Autodesk Inventor part; units mm, degrees
ref_plane "YZ Plane" through (0, 0, 0) normal (1, 0, 0) x (0, 1, 0)
ref_plane "XZ Plane" through (0, 0, 0) normal (0, 1, 0) x (-1, 0, 0)
sketch "Sketch1" plane through (0, 0, 0) normal (0, 0, 1) x (1, 0, 0)
  line L0 (-50, 20) -> (50, 20)
  line L1 (50, 20) -> (50, -20)
  line L2 (50, -20) -> (-50, -20)
  line L3 (-50, -20) -> (-50, 20)
  line L4 (-50, 20) -> (50, -20) construction
  line L5 (50, 20) -> (-50, -20) construction
  point P0 (0, 0)
  dimension "d0" = 100
  dimension "d1" = 40
extrude "Extrusion1" add sketch "Sketch1" along normal blind 20
sketch "Sketch2" plane through (0, 0, 20) normal (0, 0, 1) x (1, 0, 0)
  line L0 (-50, -20) -> (50, -20)
  line L1 (50, -20) -> (50, 20)
  line L2 (50, 20) -> (-50, 20)
  line L3 (-50, 20) -> (-50, -20)
  line L4 (-70, 0) -> (70, 0)
  line L5 (0, -28) -> (0, 28)
  line L6 (50, -20) -> (50, 20)
  line L7 (-50, 17) -> (50, 17)
  line L8 (50, 17) -> (50, 18.5)
  line L9 (50, 18.5) -> (-50, 18.5)
  line L10 (-50, 18.5) -> (-50, 17)
  line L11 (-50, 17) -> (50, 18.5) construction
  line L12 (50, 17) -> (-50, 18.5) construction
  point P0 (0, 0)
  point P1 (0, 17.75)
  dimension "d4" = 1.5
  dimension "d6" = 1.5
extrude "Extrusion2" cut sketch "Sketch2" against normal blind 17 contours L3 L9 L5 L7 | L5 L9 L1 L7
pattern_linear "Rectangular Pattern1" count 13 spacing 3 along (0, -1, 0) of "Extrusion2"
ref_plane "Work Plane1" through (0, 0, 20) normal (0, 0, 1) x (1, 0, 0)
sketch "Sketch4" plane through (0, 0, 20) normal (0, 0, 1) x (1, 0, 0)
  line L0 (0, -28) -> (0, 28)
  line L1 (50, 0.5) -> (50, -1)
  line L2 (50, 20) -> (-50, 20)
  line L3 (-50, -20) -> (50, -20)
  line L4 (-50, -4) -> (-50, -5.5)
  point P0 (0, 0)
  point P1 (44, -13)
  point P2 (-44, -13)
  dimension "d22" = 6
  dimension "d30" = 7
  dimension "d31" = 7
  dimension "d32" = 6
hole "Hole2" at (44, -13, 20) at (-44, -13, 20) direction (0, 0, -1) diameter 6.756 end through all
sketch "Sketch5" plane through (-50, 20, 0) normal (0, 1, 0) x (1, 0, 0)
  line L0 (-20, 0) -> (120, 0)
  line L1 (50, 4) -> (50, -24)
  line L2 (90.622, -3) -> (9.378, -3)
  line L3 (0, -20) -> (13, -20)
  line L4 (13, -20) -> (13, -3)
  line L5 (13, -3) -> (0, -3)
  line L6 (0, -3) -> (0, -20)
  line L7 (0, 0) -> (0, -20)
  point P0 (50, 0)
  dimension "d33" = 13
extrude "Extrusion3" cut sketch "Sketch5" against normal up to surface (40 mm away) contours L5 L2 L4 L3 L6
mirror "Mirror1" about plane through (0, 0, 0) normal (1, 0, 0) of "Extrusion3"
equation "\"d28\" = Thickness"
equation "\"BendRadius\" = Thickness"
equation "\"BendReliefWidth\" = Thickness"
equation "\"BendReliefDepth\" = 0.5 * Thickness"
equation "\"CornerReliefSize\" = 4 * Thickness"
equation "\"MinimumRemnant\" = 2 * Thickness"
equation "\"TransitionRadius\" = BendRadius"
equation "\"JacobiRadiusSize\" = BendRadius"
equation "\"GapSize\" = Thickness"
properties part number "ExternalHeatSinkandClamp"
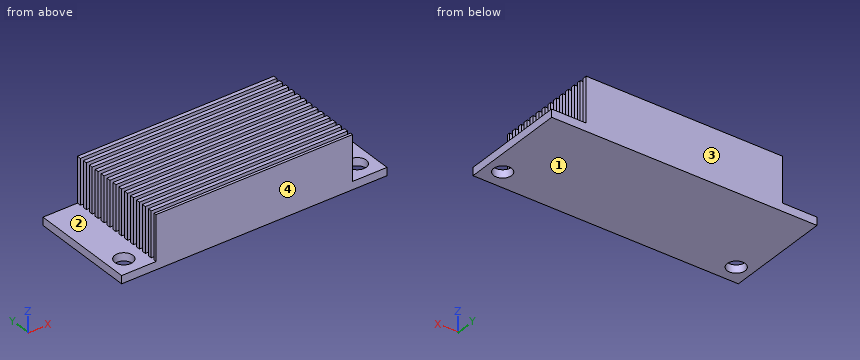
Can you work these out from the model? Positions are in its coordinate system, mm. Face numbers are marked on the shaded views. Give positions to 0.01 mm unless a question says otherwise; leave off trailing zeros. Loops run counter-clockwise (first coordinate to the right, second up) from the corner with the lowest first, then second, coordinate; pieces in that order, holes last. Notation, with made-up numbers: (-5.75, 3) -> (45.25, 3) arc R22 ccw to (45.25, 21) -> close; hole circle Ø8 at (58.5, -5). An arc over 180 degrees is marked (long way). Return JSON: item names as keys, results as strings.
Q1. We'd pull the mould along Y, two halves only. Please class the marked faces 1, 2, 3 and 4: released by +Y, released by -Y, zero draft, split by the parting line, or undercut.
Checks:
{"face 1": "zero draft", "face 2": "undercut", "face 3": "released by +Y", "face 4": "released by -Y"}
Q2. For pin 1 Ø0.8 at (y, z) = (16.5, 9) entering from -X; pin 2 Ø1.6 at (y, z) = (16.5, 13.5) entering from +X, each with a flat end and sliding along its axis, tell me the tip position at first contact or that it passes through.
Checks:
{"pin 1": "stops at x = -37", "pin 2": "stops at x = 37"}
Q3. I need wall thicknesses on probe 1 along X at (y, z) = (-13, 1.7); probe 2 along Y at (x, z) = (-44, 1.8); probe 3 along Z at (x, y) = (13, -12). Which ranges of each line are inside material? Lowest first, please.
Checks:
{"probe 1": "x = -50 to -47.38, -40.62 to 40.62, 47.38 to 50", "probe 2": "y = -20 to -16.38, -9.62 to 20", "probe 3": "z = 0 to 3"}
Q4. I want a section at B-B, the plane z = 16.75. Count the separate pieces of the cut face and the enclosed holes in it, then the cut area to 3 significant figures.
Checks:
{"separate pieces": "14", "enclosed holes": "0", "area": "1,520 mm2"}
Q5. I want a section at A-A, the plane x = 44. List the corners of the cut face in (y, z) for me.
Checks:
{"outline": "(-20, 0) -> (-16.38, 0) -> (-16.38, 3) -> (-20, 3) -> close; (-9.62, 0) -> (20, 0) -> (20, 3) -> (-9.62, 3) -> close"}
